from build123d import *

# Parameters (mm, degrees)
F0_W     = 19.05
F0_H     = 19.05
F1_DEPTH = 19.05
F2_DEPTH = 19.05
F4_W     = 19.05
F4_H     = 19.05
F5_DEPTH = 19.05
F3_W     = 19.05
F3_H     = 19.05
F6_DEPTH = 19.05
F7_DEPTH = 19.05
F8_DEPTH = 19.05


with BuildPart() as f1:
    # F0 (on Top) → F1 (new body)
    with BuildSketch(Plane.XY):
        with Locations((9.525, 9.525)):
            Rectangle(F0_W, F0_H)
    extrude(amount=F1_DEPTH)

    # F2 (add): a face of the model
    f2_faces = [f1.faces().sort_by_distance(p)[0] for p in [
        (9.525, 19.05, 9.525),
    ]]
    extrude(f2_faces, amount=F2_DEPTH)

    # F4 (on face) → F5 (join)
    with BuildSketch(Plane.YZ.offset(19.05)):
        with Locations((9.525, 9.525)):
            Rectangle(F4_W, F4_H)
    extrude(amount=F5_DEPTH)

    # F3 (on face) → F6 (join)
    with BuildSketch(Plane.XY.offset(19.05)):
        with Locations((9.525, 9.525)):
            Rectangle(F3_W, F3_H)
    extrude(amount=F6_DEPTH)

    # F7 (add): a face of the model
    f7_faces = [f1.faces().sort_by_distance(p)[0] for p in [
        (19.05, 9.525, 28.575),
    ]]
    extrude(f7_faces, amount=F7_DEPTH)

    # F8 (add): a face of the model
    f8_faces = [f1.faces().sort_by_distance(p)[0] for p in [
        (9.525, 28.575, 19.05),
    ]]
    extrude(f8_faces, amount=F8_DEPTH)


solid = f1.part
Can you work these out from the model? Positions are in its coordinate system, mm. A direction names the side the tool comes from. Round coordinates to 2 decimals unless told otherwise and drop trailing zeros. Order: outer loops, then holes, each group sorted by start corner. A loop starts at its lowest first (then second) coordinate and runs counter-clockwise, first axis right, second up. Notation, with made-up numbers: M -17.5,-24 L -13.5,-24 A12 ccw -13.5,-14 Z; hole C 89,-39.5 d3. An arc over 180 degrees is marked long. Use a Markdown table: item, result.
1) Imagine slicing it at A-A (x = 32). List the corners of the cut face in (y, z) for me.
Geometry says:
| item | result |
|---|---|
| outline | M 0,0 L 19.05,0 L 19.05,38.1 L 0,38.1 Z |
2) I'm going to push flat-ended pins straight in: P1, Ø10, axis at x = 29.5, z = 14.5, coming from the +Y side; P2, Ø6, axis at x = 23.5, y = 27.5, coming from the +Z side; P3, Ø9.5, axis at y = 25.5, z = 16.5, coming from the +X side. Where does each tip first touch, or does it pass through?
Geometry says:
| item | result |
|---|---|
| P1 | stops at y = 19.05 |
| P2 | passes through |
| P3 | stops at x = 19.05 |
3) Imagine slicing it at B-B (z = 17.5). List the corners of the cut face in (x, y) for me, then the cut area to 3 significant figures.
Geometry says:
| item | result |
|---|---|
| outline | M 0,0 L 38.1,0 L 38.1,19.05 L 19.05,19.05 L 19.05,38.1 L 0,38.1 Z |
| area | 1,090 mm² |
4) If I drill on line 1 along X through (y, z) = (30, 23.5), over which ranges is the centre line in solid material (lowest first)?
Geometry says:
| item | result |
|---|---|
| line 1 | x = 0 to 19.05 |
5) On a 3-axis mill with a long thin cutter (end or side, diameter ignored), from which of +Z, -Z, +X, -X, +Y, -Y can I reach the whole of each face in a straight line? I mean faces 1 (the face through (38.1, 9, 19)), 2 (the face through (28, 19.05, 19)). Say none if no direction works.
Geometry says:
| item | result |
|---|---|
| face 1 | +Z, -Z, +X, +Y, -Y |
| face 2 | +Z, -Z, +X, +Y |
